Verification items for this drawing (mm, ordinates from the low corner). Round coordinates to 2 decimals unless told otherwise and drop trailing zeros. Order: outer loops, then holes, each group sorted by start corner. A loop starts at its lowest first (then second) coordinate and runs counter-clockwise, first axis right, second up. Notation, with made-up numbers: (36, 45) - (67, 45) arc R23 ccw to (67, 78) - close; hole circle Ø5 at (-36, 21.5). An arc over 180 degrees is marked (long way). Use a Markdown table: item, result. Add a question column.
(1) Gauge pin test, flat ends, axial feed: P1, Ø7, axis at x = 12.5, y = 78, coming from the -Z side; P2, Ø3, axis at y = 22, z = 8, coming from the +X side; P3, Ø4, axis at y = 49.5, z = 8.5, coming from the -X side; P4, Ø2, axis at y = 69.5, z = 10.5, coming from the -X side. Record the tip position at first contact, or that the pin passes through.
(2) Section check A-A on x = 12.5. Record the boundary of the cut face in (y, z), then the cut area to 3 significant figures.
(3) Section check D-D on y = 8. Record the boundary of the cut face in (x, z).
(4) Section check B-B on y = 71.5. Record the boundary of the cut face in (x, z), then the cut area to 3 significant figures.
(5) Section check C-C on z = 4. Give the number of separate pieces and of enclosed holes in the cut face, then the cut area to 3 significant figures.
(6) Thickness scan on line 1 along Y through (x, z) = (15.75, 10.5); line 2 along Y through (x, z) = (13.5, 18.75); line 3 along X through (y, z) = (79.5, 23.25). Record the ranges inside material, lowest first. Write a range as [from, to].
(7) Mould release check, pull along X, two halves, no side actions. Record for the marked faces 1, 2 and 3: released by +X, released by -X, zero draft, split by the parting line, or undercut.
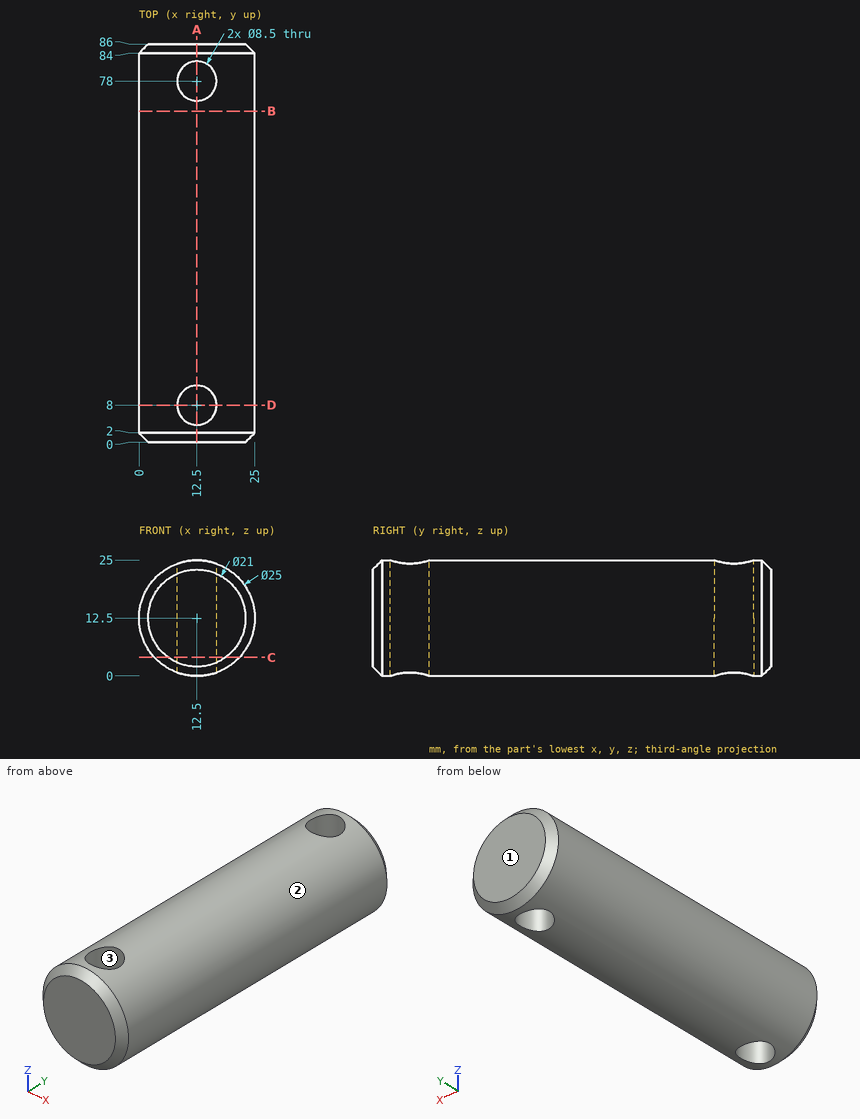
Check sheet entries:
| question | item | result |
|---|---|---|
| 1 | P1 | passes through |
| 1 | P2 | stops at x = 24.63 |
| 1 | P3 | stops at x = 0.16 |
| 1 | P4 | stops at x = 0.04 |
| 2 | outline | (0, 2) - (2, 0) - (3.75, 0) - (3.75, 25) - (2, 25) - (0, 23) - close; (12.25, 0) - (73.75, 0) - (73.75, 25) - (12.25, 25) - close; (82.25, 0) - (84, 0) - (86, 2) - (86, 23) - (84, 25) - (82.25, 25) - close |
| 2 | area | 1,720 mm2 |
| 3 | outline | (8.25, 0.74) - (8.25, 24.26) arc R12.5 ccw to start; (16.75, 0.74) arc R12.5 ccw to (16.75, 24.26) - close |
| 4 | outline | circle Ø25 at (12.5, 12.5) |
| 4 | area | 491 mm2 |
| 5 | separate pieces | 1 |
| 5 | enclosed holes | 2 |
| 5 | area | 1,450 mm2 |
| 6 | line 1 | y = [0, 5.26], [10.74, 75.26], [80.74, 86] |
| 6 | line 2 | y = [0, 3.87], [12.13, 73.87], [82.13, 86] |
| 6 | line 3 | x = [6.12, 8.52], [16.48, 18.88] |
| 7 | face 1 | zero draft |
| 7 | face 2 | split by the parting line |
| 7 | face 3 | undercut |
